Input: part model. Units: mm. Frame: model coordinates. A direction names the side the tool comes from. Give positions to 0.01 mm unless a question says otherwise; leave off trailing zeros. Loops run counter-clockwise (first coordinate to the right, second up) from the corner with the lowest first, then second, coordinate; pieces in that order, holes last. Notation, with made-up numbers: M 51,-27.5 L 100,-27.5 A19 ccw 100,4.5 Z; hole C -3.5,-34 d5. An arc over 180 degrees is marked long. Answer as a JSON object with one key per item and string values. Group by question number.
```python
from build123d import *

# Parameters (mm, degrees)
BOSS_EXTRUDE3_DEPTH = 3.175


with BuildPart() as part:
    # Model → Boss-Extrude3 (new body)
    with BuildSketch(Plane.XY):
        with BuildLine():
            Line((431.422937797, 190.288897242), (331.664437797, 190.288897242))
            ThreePointArc((331.664437797, 190.288897242), (331.484832675, 190.36329212), (331.410437797, 190.542897242))
            Line((331.410437797, 190.542897242), (331.410437797, 215.688897242))
            ThreePointArc((331.410437797, 215.688897242), (331.33604292, 215.868502364), (331.156437797, 215.942897242))
            Line((331.156437797, 215.942897242), (328.489437797, 215.942897242))
            ThreePointArc((328.489437797, 215.942897242), (328.309832675, 216.01729212), (328.235437797, 216.196897242))
            Line((328.235437797, 216.196897242), (328.235437797, 240.834897242))
            ThreePointArc((328.235437797, 240.834897242), (328.309832675, 241.014502364), (328.489437797, 241.088897242))
            Line((328.489437797, 241.088897242), (331.156437797, 241.088897242))
            ThreePointArc((331.156437797, 241.088897242), (331.33604292, 241.16329212), (331.410437797, 241.342897242))
            Line((331.410437797, 241.342897242), (331.410437797, 266.234897242))
            ThreePointArc((331.410437797, 266.234897242), (331.33604292, 266.414502364), (331.156437797, 266.488897242))
            Line((331.156437797, 266.488897242), (328.489437797, 266.488897242))
            ThreePointArc((328.489437797, 266.488897242), (328.309832675, 266.56329212), (328.235437797, 266.742897242))
            Line((328.235437797, 266.742897242), (328.235437797, 291.634897242))
            ThreePointArc((328.235437797, 291.634897242), (328.309832675, 291.814502364), (328.489437797, 291.888897242))
            Line((328.489437797, 291.888897242), (331.156437797, 291.888897242))
            ThreePointArc((331.156437797, 291.888897242), (331.33604292, 291.96329212), (331.410437797, 292.142897242))
            Line((331.410437797, 292.142897242), (331.410437797, 342.434897242))
            ThreePointArc((331.410437797, 342.434897242), (331.33604292, 342.614502364), (331.156437797, 342.688897242))
            Line((331.156437797, 342.688897242), (328.489437797, 342.688897242))
            ThreePointArc((328.489437797, 342.688897242), (328.309832675, 342.76329212), (328.235437797, 342.942897242))
            Line((328.235437797, 342.942897242), (328.235437797, 367.834897242))
            ThreePointArc((328.235437797, 367.834897242), (328.309832675, 368.014502364), (328.489437797, 368.088897242))
            Line((328.489437797, 368.088897242), (331.156437797, 368.088897242))
            ThreePointArc((331.156437797, 368.088897242), (331.33604292, 368.16329212), (331.410437797, 368.342897242))
            Line((331.410437797, 368.342897242), (331.410437797, 393.234897242))
            ThreePointArc((331.410437797, 393.234897242), (331.33604292, 393.414502364), (331.156437797, 393.488897242))
            Line((331.156437797, 393.488897242), (328.489437797, 393.488897242))
            ThreePointArc((328.489437797, 393.488897242), (328.309832675, 393.56329212), (328.235437797, 393.742897242))
            Line((328.235437797, 393.742897242), (328.235437797, 418.634897242))
            ThreePointArc((328.235437797, 418.634897242), (328.309832675, 418.814502364), (328.489437797, 418.888897242))
            Line((328.489437797, 418.888897242), (331.156437797, 418.888897242))
            ThreePointArc((331.156437797, 418.888897242), (331.33604292, 418.96329212), (331.410437797, 419.142897242))
            Line((331.410437797, 419.142897242), (331.410437797, 444.034897242))
            ThreePointArc((331.410437797, 444.034897242), (331.484832675, 444.214502364), (331.664437797, 444.288897242))
            Line((331.664437797, 444.288897242), (431.168937797, 444.288897242))
            ThreePointArc((431.168937797, 444.288897242), (431.34854292, 444.214502364), (431.422937797, 444.034897242))
            Line((431.422937797, 444.034897242), (431.422937797, 419.142897242))
            ThreePointArc((431.422937797, 419.142897242), (431.497332675, 418.96329212), (431.676937797, 418.888897242))
            Line((431.676937797, 418.888897242), (434.343937797, 418.888897242))
            ThreePointArc((434.343937797, 418.888897242), (434.52354292, 418.814502364), (434.597937797, 418.634897242))
            Line((434.597937797, 418.634897242), (434.597937797, 393.742897242))
            ThreePointArc((434.597937797, 393.742897242), (434.52354292, 393.56329212), (434.343937797, 393.488897242))
            Line((434.343937797, 393.488897242), (431.676937797, 393.488897242))
            ThreePointArc((431.676937797, 393.488897242), (431.497332675, 393.414502364), (431.422937797, 393.234897242))
            Line((431.422937797, 393.234897242), (431.422937797, 368.342897242))
            ThreePointArc((431.422937797, 368.342897242), (431.497332675, 368.16329212), (431.676937797, 368.088897242))
            Line((431.676937797, 368.088897242), (434.343937797, 368.088897242))
            ThreePointArc((434.343937797, 368.088897242), (434.52354292, 368.014502364), (434.597937797, 367.834897242))
            Line((434.597937797, 367.834897242), (434.597937797, 342.942897242))
            ThreePointArc((434.597937797, 342.942897242), (434.52354292, 342.76329212), (434.343937797, 342.688897242))
            Line((434.343937797, 342.688897242), (431.676937797, 342.688897242))
            ThreePointArc((431.676937797, 342.688897242), (431.497332675, 342.614502364), (431.422937797, 342.434897242))
            Line((431.422937797, 342.434897242), (431.422937797, 292.142897242))
            ThreePointArc((431.422937797, 292.142897242), (431.497332675, 291.96329212), (431.676937797, 291.888897242))
            Line((431.676937797, 291.888897242), (434.343937797, 291.888897242))
            ThreePointArc((434.343937797, 291.888897242), (434.52354292, 291.814502364), (434.597937797, 291.634897242))
            Line((434.597937797, 291.634897242), (434.597937797, 266.742897242))
            ThreePointArc((434.597937797, 266.742897242), (434.52354292, 266.56329212), (434.343937797, 266.488897242))
            Line((434.343937797, 266.488897242), (431.676937797, 266.488897242))
            ThreePointArc((431.676937797, 266.488897242), (431.497332675, 266.414502364), (431.422937797, 266.234897242))
            Line((431.422937797, 266.234897242), (431.422937797, 241.342897242))
            ThreePointArc((431.422937797, 241.342897242), (431.497332675, 241.16329212), (431.676937797, 241.088897242))
            Line((431.676937797, 241.088897242), (434.343937797, 241.088897242))
            ThreePointArc((434.343937797, 241.088897242), (434.52354292, 241.014502364), (434.597937797, 240.834897242))
            Line((434.597937797, 240.834897242), (434.597937797, 215.942897242))
            ThreePointArc((434.597937797, 215.942897242), (434.52354292, 215.76329212), (434.343937797, 215.688897242))
            Line((434.343937797, 215.688897242), (431.676937797, 215.688897242))
            ThreePointArc((431.676937797, 215.688897242), (431.497332675, 215.614502364), (431.422937797, 215.434897242))
            Line((431.422937797, 215.434897242), (431.422937797, 190.288897242))
        make_face()
        with BuildLine():
            Line((382.786560027, 297.127371964), (411.075896543, 207.115846687))
            ThreePointArc((411.075896543, 207.115846687), (410.606562601, 204.285309273), (408.046966492, 202.988897242))
            Line((408.046966492, 202.988897242), (357.094405319, 202.988897242))
            ThreePointArc((357.094405319, 202.988897242), (354.550237774, 204.264466668), (354.050329968, 207.066244326))
            Line((354.050329968, 207.066244326), (380.739668991, 297.102568741))
            ThreePointArc((380.739668991, 297.102568741), (381.123130271, 297.75765158), (381.766901137, 298.15981467))
            ThreePointArc((381.766901137, 298.15981467), (382.401598049, 297.766914662), (382.786560027, 297.127371964))
        make_face(mode=Mode.SUBTRACT)
        with BuildLine():
            Line((394.40551129, 298.238897242), (415.547937797, 298.238897242))
            ThreePointArc((415.547937797, 298.238897242), (417.793001827, 297.308961272), (418.722937797, 295.063897242))
            Line((418.722937797, 295.063897242), (418.722937797, 224.025344178))
            ThreePointArc((418.722937797, 224.025344178), (416.005554119, 220.88349563), (412.504851308, 223.119667846))
            Line((412.504851308, 223.119667846), (391.362427311, 294.158212475))
            ThreePointArc((391.362427311, 294.158212475), (391.860302641, 296.961932524), (394.40551129, 298.238897242))
        make_face(mode=Mode.SUBTRACT)
        with BuildLine():
            Line((354.71801129, 431.588897242), (408.046966492, 431.588897242))
            ThreePointArc((408.046966492, 431.588897242), (410.606562601, 430.292485211), (411.075896543, 427.461947797))
            Line((411.075896543, 427.461947797), (382.786560027, 337.45042252))
            ThreePointArc((382.786560027, 337.45042252), (382.211388986, 336.646599187), (381.272095002, 336.338897242))
            Line((381.272095002, 336.338897242), (379.992498353, 336.338897242))
            ThreePointArc((379.992498353, 336.338897242), (379.043481575, 336.653792274), (378.470956978, 337.473552796))
            Line((378.470956978, 337.473552796), (351.674924794, 427.508220933))
            ThreePointArc((351.674924794, 427.508220933), (352.172805279, 430.311936061), (354.71801129, 431.588897242))
        make_face(mode=Mode.SUBTRACT)
        with BuildLine():
            Line((418.722937797, 403.356536927), (418.722937797, 339.513897242))
            ThreePointArc((418.722937797, 339.513897242), (417.793001827, 337.268833212), (415.547937797, 336.338897242))
            Line((415.547937797, 336.338897242), (396.623155319, 336.338897242))
            ThreePointArc((396.623155319, 336.338897242), (394.078987861, 337.614466553), (393.579079886, 340.416244049))
            Line((393.579079886, 340.416244049), (412.503864616, 404.25889133))
            ThreePointArc((412.503864616, 404.25889133), (416.003839459, 406.498634741), (418.722937797, 403.356536927))
        make_face(mode=Mode.SUBTRACT)
        with BuildLine():
            Line((350.314367848, 400.447983443), (369.165896543, 340.465846687))
            ThreePointArc((369.165896543, 340.465846687), (368.696562601, 337.635309273), (366.136966492, 336.338897242))
            Line((366.136966492, 336.338897242), (347.285437797, 336.338897242))
            ThreePointArc((347.285437797, 336.338897242), (345.040373767, 337.268833212), (344.110437797, 339.513897242))
            Line((344.110437797, 339.513897242), (344.110437797, 399.496038941))
            ThreePointArc((344.110437797, 399.496038941), (346.803894766, 402.634304431), (350.314367848, 400.447983443))
        make_face(mode=Mode.SUBTRACT)
        with BuildLine():
            Line((369.165896543, 294.111947797), (350.314367848, 234.129811041))
            ThreePointArc((350.314367848, 234.129811041), (346.803894766, 231.943490053), (344.110437797, 235.081755542))
            Line((344.110437797, 235.081755542), (344.110437797, 295.063897242))
            ThreePointArc((344.110437797, 295.063897242), (345.040373767, 297.308961272), (347.285437797, 298.238897242))
            Line((347.285437797, 298.238897242), (366.136966492, 298.238897242))
            ThreePointArc((366.136966492, 298.238897242), (368.696562601, 296.942485211), (369.165896543, 294.111947797))
        make_face(mode=Mode.SUBTRACT)
    extrude(amount=BOSS_EXTRUDE3_DEPTH)


solid = part.part
```
1. Section B-B (x = 385). Output: boundary loops of the cut face in (y, z) (3 decimals), then the cut area to 3 significant figures.
2. Reachability of faces 4 (the flat face through (382, 319, 0)), 5 (the flat face through (359.6, 370.9, 1.6)) from +Z, -Z, +X, -X, +Y, -Y: full face, straight path, thin tool, end or side. Return the list, or none.
3. First-contact query: P1, Ø1.3, axis at x = 329.5, z = 2, coming from the +Y side; P2, Ø1.6, axis at y = 248, z = 2, coming from the -X side; P3, Ø1.3, axis at x = 329, z = 1, coming from the -Y side. Flat tips, straight axial feed; report the tip coordinate or a pass-through.
4. Section C-C (z = 1.95). Count the separate pieces of the cut face and the enclosed holes in it, then the cut area to 3 significant figures.
5. Section A-A (y = 278.5). Output: boundary loops of the cut face in (x, z) (3 decimals).
6. Mould query, pull axis Y, two halves, no side actions, for faces 1 (the flat face through (382, 319, 3.175)), 2 (the flat face through (402.91, 371.89, 1.57)), 3 (the flat face through (397.13, 383.09, 1.57)). Classes: pulls with the +Y half, pulls with the -Y half, needs draft (parallel to the pull), parting line crosses it, or undercut.
7. Material intervals for L1, parallel to X at y = 294, z = 1.05; L2, parallel to X at y = 227, z = 1.45; L3, parallel to X at y = 277.5, z = 1.75 (3 decimals), sorted ascending.
8. Section D-D (y = 371). Output: boundary loops of the cut face in (x, z) (3 decimals), then the cut area to 3 significant figures.
Geometry results:
{
 "1": {"outline": "M 190.289,0 L 202.989,0 L 202.989,3.175 L 190.289,3.175 Z; M 290.085,0 L 344.493,0 L 344.493,3.175 L 290.085,3.175 Z; M 431.589,0 L 444.289,0 L 444.289,3.175 L 431.589,3.175 Z", "area": "253 mm2"},
 "2": {"face 4": "-Z, +X, -X, +Y, -Y", "face 5": "+Z, -Z"},
 "3": {"P1": "y = 418.89", "P2": "x = 331.41", "P3": "y = 215.94"},
 "4": {"separate pieces": "1", "enclosed holes": "6", "area": "15,500 mm2"},
 "5": {"outline": "M 328.235,0 L 344.11,0 L 344.11,3.175 L 328.235,3.175 Z; M 364.259,0 L 375.225,0 L 375.225,3.175 L 364.259,3.175 Z; M 388.641,0 L 396.023,0 L 396.023,3.175 L 388.641,3.175 Z; M 418.723,0 L 434.598,0 L 434.598,3.175 L 418.723,3.175 Z"},
 "6": {"face 1": "needs draft", "face 2": "undercut", "face 3": "undercut"},
 "7": {"L1": "331.41 to 344.11, 369.13 to 379.82, 383.77 to 391.41, 418.72 to 431.42", "L2": "328.24 to 359.96, 404.83 to 411.35, 418.72 to 434.6", "L3": "328.235 to 344.11, 363.945 to 374.929, 388.955 to 396.32, 418.723 to 434.598"},
 "8": {"outline": "M 331.41,0 L 344.11,0 L 344.11,3.175 L 331.41,3.175 Z; M 359.569,0 L 368.493,0 L 368.493,3.175 L 359.569,3.175 Z; M 393.331,0 L 402.645,0 L 402.645,3.175 L 393.331,3.175 Z; M 418.723,0 L 431.423,0 L 431.423,3.175 L 418.723,3.175 Z", "area": "139 mm2"}
}
